```python
from build123d import *

# Parameters (mm, degrees)
F0_R     = 10
F1_DEPTH = 15


with BuildPart() as f1:
    # F0 (on Front) → F1 (new body)
    with BuildSketch(Plane.XZ):
        Polygon((-372.5, 80), (-412.5, 80), (-412.5, -80), (-332.5, -80), (332.5, -80), (412.5, -80), (412.5, 80), (372.5, 80), (372.5, 0), (357.5, 0), (357.5, 80), (297.5, 80), (297.5, 48), (257.5, 48), (257.5, 80), (107.5, 80), (107.5, 48), (67.5, 48), (67.5, 80), (7.5, 80), (7.5, 0), (-7.5, 0), (-7.5, 80), (-67.5, 80), (-67.5, 48), (-107.5, 48), (-107.5, 80), (-257.5, 80), (-257.5, 48), (-297.5, 48), (-297.5, 80), (-357.5, 80), (-357.5, 0), (-372.5, 0), align=None)
        with Locations((-277.5, 0)):
            Circle(F0_R, mode=Mode.SUBTRACT)
        with Locations((-182.5, 0)):
            Circle(F0_R, mode=Mode.SUBTRACT)
        with Locations((-87.5, 0)):
            Circle(F0_R, mode=Mode.SUBTRACT)
        with Locations((87.5, 0)):
            Circle(F0_R, mode=Mode.SUBTRACT)
        with Locations((182.5, 0)):
            Circle(F0_R, mode=Mode.SUBTRACT)
        with Locations((277.5, 0)):
            Circle(F0_R, mode=Mode.SUBTRACT)
    extrude(amount=F1_DEPTH)


solid = f1.part
```
Source: CAD feature listing. Evaluate the final solid. Frame: model axes, mm. A direction names the side the tool comes from. Coordinates: 2 decimals unless noted, no trailing zeros. Loops run counter-clockwise (first coordinate to the right, second up) from the corner with the lowest first, then second, coordinate; pieces in that order, holes last. Notation, with made-up numbers: M -26.5,-15.75 L 7.5,-15.75 A16 ccw 7.5,11.25 Z; hole C 24.25,0.25 d10. An arc over 180 degrees is marked long. Use a Markdown table: item, result. Add a question column.
Q1. First-contact query: pin 1 (6 mm diameter, centred on x = 166, z = -30.5, fed in from +Y); pin 2 (7.5 mm diameter, centred on x = 362, y = -10, fed in from +Z); pin 3 (7.5 mm diameter, centred on x = 285, y = -7.5, fed in from +Z). Flat tips, straight axial feed; report the tip coordinate or a pass-through.
Q2. Material intervals for L1, parallel to X at y = -1, z = 19.5; L2, parallel to Z at x = 277.5, y = -8; L3, parallel to Z at x = -182.5, y = -4.5, sorted ascending.
Q3. Section query C-C, the plane x = -182.5. Return loops of the section in (y, z).
Q4. Draft query along Z for faces 1 (the flat face through (-6, -7, -80)), 2 (the flat face through (-357.5, -7, 41)), 3 (the cylindrical face through (-285.44, -7.4, -6.08)), 4 (the flat face through (184, -7, 80)). Return one class per face: pulls with the +Z half, pulls with the -Z half, needs draft (parallel to the pull), parting line crosses it, or undercut.
Q5. Section query A-A, the plane x = -87.5. Return loops of the section in (y, z), and give its area (3 significant figures).
Q6. Section query B-B, the plane y = -9.75. State how many separate pieces and enclosed holes the cut face has, and give its area (3 significant figures).
Q7. Access query for faces 5 (the cylindrical face through (77.51, -7.4, 0.44)), 6 (the flat face through (-297.5, -7, 64)). Directions: +Z, -Z, +X, -X, +Y, -Y. A direction counts if a zero-diameter tool reaches every point of the face in a straight line with its end or side. Return the directions, or none.
Result:
| question | item | result |
|---|---|---|
| 1 | pin 1 | stops at y = 0 |
| 1 | pin 2 | stops at z = 0 |
| 1 | pin 3 | stops at z = 48 |
| 2 | L1 | x = -412.5 to -372.5, -357.5 to -7.5, 7.5 to 357.5, 372.5 to 412.5 |
| 2 | L2 | z = -80 to -10, 10 to 48 |
| 2 | L3 | z = -80 to -10, 10 to 80 |
| 3 | outline | M -15,-80 L 0,-80 L 0,-10 L -15,-10 Z; M -15,10 L 0,10 L 0,80 L -15,80 Z |
| 4 | face 1 | pulls with the -Z half |
| 4 | face 2 | needs draft |
| 4 | face 3 | undercut |
| 4 | face 4 | pulls with the +Z half |
| 5 | outline | M -15,-80 L 0,-80 L 0,-10 L -15,-10 Z; M -15,10 L 0,10 L 0,48 L -15,48 Z |
| 5 | area | 1,620 mm2 |
| 6 | separate pieces | 1 |
| 6 | enclosed holes | 6 |
| 6 | area | 121,000 mm2 |
| 7 | face 5 | +Y, -Y |
| 7 | face 6 | +Z, +Y, -Y |
